The listing builds one solid part. Answer for the finished solid, in the listing's coordinates (mm). Give positions to 0.01 mm unless a question says otherwise; leave off trailing zeros. Order: outer loops, then holes, each group sorted by start corner. A loop starts at its lowest first (then second) coordinate and runs counter-clockwise, first axis right, second up. Notation, with made-up numbers: M 12,3.25 L 16,3.25 A19 cw 16,21.25 Z; hole C 46,-36.5 d7. An arc over 180 degrees is marked long. Answer as a JSON object with one key per item and string values. Group by question number.
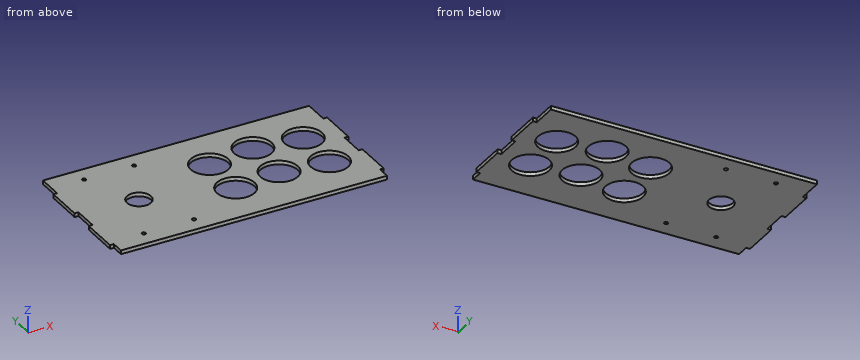
```python
from build123d import *

# Parameters (mm, degrees)
F0_R     = 1.5
F0_R_2   = 14.85
F0_R_3   = 9.5
F0_W     = 3
F0_H     = 30
F1_DEPTH = 3


with BuildPart() as f1:
    # F0 (on Top) → F1 (new body)
    with BuildSketch(Plane.XY):
        Polygon((105, 55), (-105, 55), (-105, 35), (-105, 5), (-105, -15), (-105, -45), (-105, -55), (105, -55), (105, -45), (105, -15), (105, 5), (105, 35), align=None)
        with Locations((-79.75, -42.25)):
            Circle(F0_R, mode=Mode.SUBTRACT)
        with Locations((-40.25, -42.25)):
            Circle(F0_R, mode=Mode.SUBTRACT)
        with Locations((6, -18.5)):
            Circle(F0_R_2, mode=Mode.SUBTRACT)
        with Locations((43, -13.5)):
            Circle(F0_R_2, mode=Mode.SUBTRACT)
        with Locations((80, -18.5)):
            Circle(F0_R_2, mode=Mode.SUBTRACT)
        with Locations((-60, 0)):
            Circle(F0_R_3, mode=Mode.SUBTRACT)
        with Locations((-79.75, 42.25)):
            Circle(F0_R, mode=Mode.SUBTRACT)
        with Locations((-40.25, 42.25)):
            Circle(F0_R, mode=Mode.SUBTRACT)
        with Locations((6, 18.5)):
            Circle(F0_R_2, mode=Mode.SUBTRACT)
        with Locations((43, 23.5)):
            Circle(F0_R_2, mode=Mode.SUBTRACT)
        with Locations((80, 18.5)):
            Circle(F0_R_2, mode=Mode.SUBTRACT)
        with Locations((-106.5, 20)):
            Rectangle(F0_W, F0_H)
        with Locations((106.5, 20)):
            Rectangle(F0_W, F0_H)
        with Locations((-106.5, -30)):
            Rectangle(F0_W, F0_H)
        with Locations((106.5, -30)):
            Rectangle(F0_W, F0_H)
    extrude(amount=F1_DEPTH)


solid = f1.part
```
Item 1: Section D-D (x = -3) is taken. Determine the outline of the cut face in (y, z), and give its area (3 significant figures).
Item 2: Section A-A (x = 80) is taken. Determine the outline of the cut face in (y, z).
Item 3: Section C-C (y = 18.5) is taken. Determine the outline of the cut face in (x, z), and give its area (3 significant figures).
Item 4: Consider probe 1 along Y at (x, z) = (6, 1.85); probe 2 along Y at (x, z) = (43, 1.85); probe 3 along X at (y, z) = (43, 0.8). Determine where each line is inside the solid, lowest interval first. Write a range as from..to.
Item 5: Flat-ended cylindrical pins translate along their axes: P1, Ø1.5, axis at x = 106.5, z = 2, coming from the -Y side; P2, Ø1.5, axis at y = -50, z = 2, coming from the +X side. Find the tip coordinate at first contact, or state that the pin passes through.
Item 6: Section B-B (z = 2.3) is taken. Count the separate pieces of the cut face and the enclosed holes in it, and give its area (3 significant figures).
Values found:
{
 "1": {"outline": "M -55,0 L -30.31,0 L -30.31,3 L -55,3 Z; M -6.69,0 L 6.69,0 L 6.69,3 L -6.69,3 Z; M 30.31,0 L 55,0 L 55,3 L 30.31,3 Z", "area": "188 mm^2"},
 "2": {"outline": "M -55,0 L -33.35,0 L -33.35,3 L -55,3 Z; M -3.65,0 L 3.65,0 L 3.65,3 L -3.65,3 Z; M 33.35,0 L 55,0 L 55,3 L 33.35,3 Z"},
 "3": {"outline": "M -108,0 L -8.85,0 L -8.85,3 L -108,3 Z; M 20.85,0 L 29.02,0 L 29.02,3 L 20.85,3 Z; M 56.98,0 L 65.15,0 L 65.15,3 L 56.98,3 Z; M 94.85,0 L 108,0 L 108,3 L 94.85,3 Z", "area": "386 mm^2"},
 "4": {"probe 1": "y = -55..-33.35, -3.65..3.65, 33.35..55", "probe 2": "y = -55..-28.35, 1.35..8.65, 38.35..55", "probe 3": "x = -105..-81.05, -78.45..-41.55, -38.95..105"},
 "5": {"P1": "stops at y = -45", "P2": "stops at x = 105"},
 "6": {"separate pieces": "1", "enclosed holes": "11", "area": "19,000 mm^2"}
}
